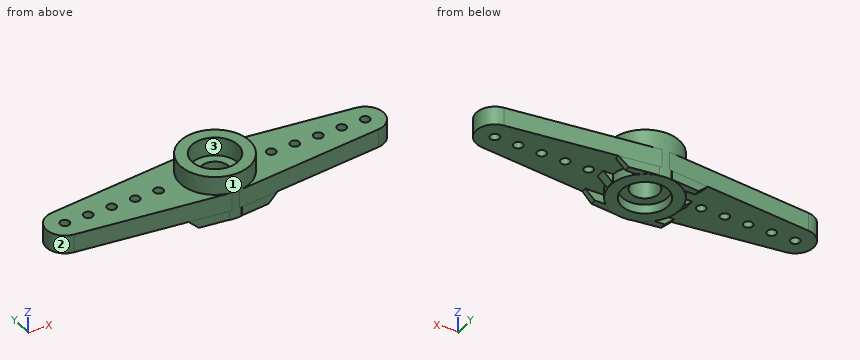
```python
from build123d import *

# Parameters (mm, degrees)
CROQUIS1_R              = 0.5
CROQUIS1_R_2            = 2
CROQUIS1_R_3            = 3.75
CROQUIS1_R_4            = 2.5
CROQUIS1_R_5            = 1.5
SALIENTE_EXTRUIR1_DEPTH = 1
SALIENTE_EXTRUIR2_START = -2
CROQUIS1_3_R            = 3.75
CROQUIS1_3_R_2          = 2.5
SALIENTE_EXTRUIR2_DEPTH = 1
SALIENTE_EXTRUIR3_START = 1
CROQUIS1_4_R            = 3.75
CROQUIS1_4_R_2          = 2.5
SALIENTE_EXTRUIR3_DEPTH = 2
SALIENTE_EXTRUIR5_DEPTH = 0.5
SALIENTE_EXTRUIR6_START = 3.75
SALIENTE_EXTRUIR6_DEPTH = 1
SALIENTE_EXTRUIR7_START = -3.75
SALIENTE_EXTRUIR7_DEPTH = 1
CORTAR_EXTRUIR1_DEPTH   = 3


with BuildPart() as part:
    # Croquis1 → Saliente-Extruir1 (new, symmetric)
    with BuildSketch(Plane.XY):
        with BuildLine():
            ThreePointArc((-0.410156, -3.727502), (-3.75, 0), (-0.410156, 3.727502))
            Line((-0.410156, 3.727502), (-16.21875, 1.988001))
            ThreePointArc((-16.21875, 1.988001), (-14.665365, 1.489547), (-14, 0))
            ThreePointArc((-14, 0), (-14.665365, -1.489547), (-16.21875, -1.988001))
            Line((-16.21875, -1.988001), (-0.410156, -3.727502))
        make_face()
        with BuildLine():
            ThreePointArc((-13, 0), (-13.5, -0.5), (-14, 0))
            ThreePointArc((-14, 0), (-13.5, 0.5), (-13, 0))
        make_face(mode=Mode.SUBTRACT)
        with Locations((-11, 0)):
            Circle(CROQUIS1_R, mode=Mode.SUBTRACT)
        with Locations((-8.5, 0)):
            Circle(CROQUIS1_R, mode=Mode.SUBTRACT)
        with Locations((-6, 0)):
            Circle(CROQUIS1_R, mode=Mode.SUBTRACT)
        with Locations((-16, 0)):
            Circle(CROQUIS1_R_2)
        with Locations((-16, 0)):
            Circle(CROQUIS1_R, mode=Mode.SUBTRACT)
        Circle(CROQUIS1_R_3)
        Circle(CROQUIS1_R_4, mode=Mode.SUBTRACT)
        Circle(CROQUIS1_R_4)
        Circle(CROQUIS1_R_5, mode=Mode.SUBTRACT)
        with BuildLine():
            Line((16.21875, 1.988001), (0.410156, 3.727502))
            ThreePointArc((0.410156, 3.727502), (2.7929, 2.50244), (3.75, 0))
            ThreePointArc((3.75, 0), (2.7929, -2.50244), (0.410156, -3.727502))
            Line((0.410156, -3.727502), (16.21875, -1.988001))
            ThreePointArc((16.21875, -1.988001), (14.665365, -1.489547), (14, 0))
            ThreePointArc((14, 0), (14.665365, 1.489547), (16.21875, 1.988001))
        make_face()
        with Locations((6, 0)):
            Circle(CROQUIS1_R, mode=Mode.SUBTRACT)
        with Locations((8.5, 0)):
            Circle(CROQUIS1_R, mode=Mode.SUBTRACT)
        with Locations((11, 0)):
            Circle(CROQUIS1_R, mode=Mode.SUBTRACT)
        with Locations((13.5, 0)):
            Circle(CROQUIS1_R, mode=Mode.SUBTRACT)
        with Locations((16, 0)):
            Circle(CROQUIS1_R_2)
        with Locations((16, 0)):
            Circle(CROQUIS1_R, mode=Mode.SUBTRACT)
    extrude(amount=SALIENTE_EXTRUIR1_DEPTH, both=True)

    # Croquis1<3> → Saliente-Extruir2 (add)
    with BuildSketch(Plane.XY.offset(SALIENTE_EXTRUIR2_START)):
        with Locations(Location((0, 0, 0), (0, 0, 263.720712))):
            Circle(CROQUIS1_3_R)
        Circle(CROQUIS1_3_R_2, mode=Mode.SUBTRACT)
    extrude(amount=SALIENTE_EXTRUIR2_DEPTH)

    # Croquis1<4> → Saliente-Extruir3 (add)
    with BuildSketch(Plane.XY.offset(SALIENTE_EXTRUIR3_START)):
        Circle(CROQUIS1_4_R)
        Circle(CROQUIS1_4_R_2, mode=Mode.SUBTRACT)
    extrude(amount=SALIENTE_EXTRUIR3_DEPTH)

    # Croquis3 → Saliente-Extruir5 (add, symmetric)
    with BuildSketch(Plane(origin=(0, 0, 0), x_dir=(1, 0, 0), z_dir=(0, 1, 0))):
        Polygon((-4.75, 1), (-3.678391, 2), (-3.678391, 1), align=None)
        Polygon((3.678391, 1), (4.75, 1), (3.678391, 2), align=None)
    extrude(amount=SALIENTE_EXTRUIR5_DEPTH, both=True)

    # Croquis4 → Saliente-Extruir6 (add)
    with BuildSketch(Plane(origin=(0, 0, 0), x_dir=(1, 0, 0), z_dir=(0, 1, 0)).offset(SALIENTE_EXTRUIR6_START)):
        Polygon((-4.75, 1), (-0.650356, 1), (-0.650356, 1.964422), (-3.716517, 1.964422), align=None)
        Polygon((0.650356, 1.964422), (0.650356, 1), (4.75, 1), (3.716517, 1.964422), align=None)
    extrude(amount=-SALIENTE_EXTRUIR6_DEPTH)

    # Croquis4<2> → Saliente-Extruir7 (add)
    with BuildSketch(Plane(origin=(0, 0, 0), x_dir=(1, 0, 0), z_dir=(0, 1, 0)).offset(SALIENTE_EXTRUIR7_START)):
        Polygon((-4.75, 1), (-0.650356, 1), (-0.650356, 1.964422), (-3.716517, 1.964422), align=None)
        Polygon((0.650356, 1.964422), (0.650356, 1), (4.75, 1), (3.716517, 1.964422), align=None)
    extrude(amount=SALIENTE_EXTRUIR7_DEPTH)

    # Croquis5 → Cortar-Extruir1 (cut)
    with BuildSketch(Plane.XY.offset(-1)):
        Polygon((0.650356, -3.75), (4.75, -3.75), (4.75, -3.249967), (0.650356, -3.701072), align=None)
        Polygon((-0.650356, -3.701072), (-0.650356, -3.75), (-4.75, -3.75), (-4.75, -3.249967), align=None)
        Polygon((-4.75, 3.75), (-4.75, 3.249967), (-0.650356, 3.701072), (-0.650356, 3.75), align=None)
        Polygon((0.650356, 3.701072), (0.650356, 3.75), (4.75, 3.75), (4.75, 3.249967), align=None)
    extrude(amount=-CORTAR_EXTRUIR1_DEPTH, mode=Mode.SUBTRACT)


solid = part.part
```
Verification items for the finished model (mm, model axes). Face numbers are marked on the shaded views. A direction names the side the tool comes from. Give positions to 0.01 mm unless a question says otherwise; leave off trailing zeros. Loops run counter-clockwise (first coordinate to the right, second up) from the corner with the lowest first, then second, coordinate; pieces in that order, holes last.
1. Section check D-D, the plane y = 0. Count the separate pieces of the cut face and the enclosed holes in it, then the cut area to 3 significant figures.
2. Section check A-A, the plane x = 0. Enter the section's corners in (y, z), then the cut area to 3 significant figures.
3. Go/stop test with flat-tipped pins: pin 1 Ø1.1 at (x, z) = (3.5, -1.5) entering from +Y; pin 2 Ø0.5 at (x, z) = (-4.5, -1.5) entering from -Y; pin 3 Ø2.5 at (x, y) = (0, 0) entering from +Z; pin 4 Ø0.8 at (x, z) = (-4, -1.5) entering from -Y. Record where each tip stops, or that it passes through.
4. Section check C-C, the plane x = -6. Enter the section's corners in (y, z).
5. Thickness scan on line 1 (Y direction, x = 0, z = -0.5); line 2 (Y direction, x = -4.5, z = -1.1); line 3 (Z direction, x = 7, y = 0). Record the ranges inside material, lowest first.
6. Section check B-B, the plane z = 1.7. Enter the section's corners in (x, y), then the cut area to 3 significant figures.
7. Set-up check for the marked faces 1, 2 and 3: record each of +Z, -Z, +X, -X, +Y, -Y from which the full face is reachable in a straight line by a thin tool's end or side.
Geometry says:
1. separate pieces: 12
1. enclosed holes: 0
1. area: 54.4 mm2
2. outline: (-3.75, -2) - (-2.5, -2) - (-2.5, -1) - (-1.5, -1) - (-1.5, 1) - (-2.5, 1) - (-2.5, 3) - (-3.75, 3) - close; (1.5, -1) - (2.5, -1) - (2.5, -2) - (3.75, -2) - (3.75, 3) - (2.5, 3) - (2.5, 1) - (1.5, 1) - close
2. area: 16.5 mm2
3. pin 1: stops at y = 3.45
3. pin 2: stops at y = -3.3
3. pin 3: passes through
3. pin 4: stops at y = -3.38
4. outline: (-3.11, -1) - (-0.5, -1) - (-0.5, 1) - (-3.11, 1) - close; (0.5, -1) - (3.11, -1) - (3.11, 1) - (0.5, 1) - close
5. line 1: y = -3.75 to -1.5, 1.5 to 3.75
5. line 2: y = -3.28 to -2.75, -0.5 to 0.5, 2.75 to 3.28
5. line 3: z = -1 to 1
6. outline: circle Ø7.5 at (0, 0); hole circle Ø5 at (0, 0)
6. area: 24.5 mm2
7. face 1: none
7. face 2: +Z, -Z, -X
7. face 3: +Z
